Verification items for the finished model (mm, model axes). Give positions to 0.01 mm unless a question says otherwise; leave off trailing zeros. Order: outer loops, then holes, each group sorted by start corner. A loop starts at its lowest first (then second) coordinate and runs counter-clockwise, first axis right, second up.
(1) Scan lines: L1, parallel to X at y = 0.5, z = 17; L2, parallel to Y at x = -9, z = 109; L3, parallel to Y at x = -18, z = 23. Record each from-to range of solid material in increasing order.
(2) Sectioned sample at A-A on z = 123. Record the cut outline in (x, y), plus the area to 3 significant figures.
(3) Sectioned sample at C-C on y = 5.5. Record the cut outline in (x, z), plus the area to 3 significant figures.
(4) Sectioned sample at B-B on x = 7. Record the cut outline in (y, z).
(5) Gauge pin test, flat ends, axial feed: pin 1 (6 mm diameter, centred on x = 5, y = 24, fed in from +Z); pin 2 (9.5 mm diameter, centred on x = -3.5, z = 46, fed in from +Y); pin 3 (2 mm diameter, centred on y = 10, z = 128.5, fed in from -X). Record the tip position at first contact, or that the pin passes through.
```python
from build123d import *

# Parameters (mm, degrees)
EXTRUDE_1_DEPTH = 144
SKETCH_2_R      = 1
EXTRUDE_2_DEPTH = 20


with BuildPart() as part:
    # 스케치1 → 보스-돌출1 (new body)
    with BuildSketch(Plane.XY):
        with BuildLine():
            Line((-16, -10), (16, -10))
            ThreePointArc((16, -10), (25.405398904, -3.396832561), (22.38971305, 7.69230571))
            Line((22.38971305, 7.69230571), (16.000004032, 13))
            Line((16.000004032, 13), (-16, 13))
            Line((-16, 13), (-22.389710664, 7.692307692))
            ThreePointArc((-22.389710664, 7.692307692), (-25.405399431, -3.396831102), (-16, -10))
        make_face()
    extrude(amount=EXTRUDE_1_DEPTH)

    # 스케치2 → 보스-돌출2 (add)
    with BuildSketch(Plane(origin=(0, 13, 0), x_dir=(1, 0, 0), z_dir=(0, 1, 0))):
        with Locations(Location((-3, -1.5, 0), (0, 0, 90))):
            Circle(SKETCH_2_R)
        with Locations(Location((0, -1.5, 0), (0, 0, 90))):
            Circle(SKETCH_2_R)
        with Locations(Location((3, -1.5, 0), (0, 0, 90))):
            Circle(SKETCH_2_R)
    extrude(amount=EXTRUDE_2_DEPTH)


solid = part.part
```
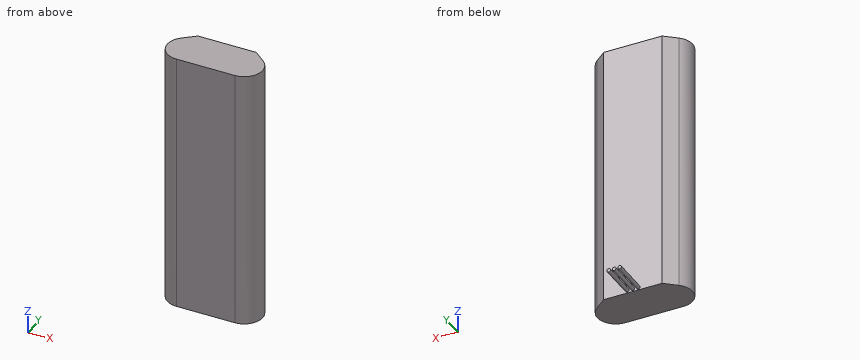
Ans:
1. L1: x = -25.99 to 25.99
1. L2: y = -10 to 13
1. L3: y = -9.8 to 11.34
2. outline: (-22.39, 7.69) arc R10 ccw to (-16, -10) - (16, -10) arc R10 ccw to (22.39, 7.69) - (16, 13) - (-16, 13) - close
2. area: 1,060 mm2
3. outline: (-24.35, 0) - (24.35, 0) - (24.35, 144) - (-24.35, 144) - close
3. area: 7,010 mm2
4. outline: (-10, 0) - (13, 0) - (13, 144) - (-10, 144) - close
5. pin 1: stops at z = 2.5
5. pin 2: stops at y = 13
5. pin 3: stops at x = -20.82
